Part model, mm, in its own coordinate system. Face numbers are marked on the shaded views. A direction names the side the tool comes from. Coordinates: 2 decimals unless noted, no trailing zeros. Loops run counter-clockwise (first coordinate to the right, second up) from the corner with the lowest first, then second, coordinate; pieces in that order, holes last. Notation, with made-up numbers: (29, 60) -> (52, 60) arc R22 cw to (52, 99) -> close; hole circle Ø5 at (-15.5, 8). An arc over 180 degrees is marked (long way). One line per question, with ' | ' between items. Start each with the question number.
1) Two-plate mould, pull along X, no slides. Class the marked faces 4, 5, 6 and 7: released by +X, released by -X, zero draft, split by the parting line, or undercut.
2) 3-axis set-ups, long thin cutter, end or side, ignore diameter. For the marked faces 1, 2 and 3: which of +Z, -Z, +X, -X, +Y, -Y reach the whole face in a straight line?
3) Cut at A-A (z = 45). List the corners of the cut face in (x, y), plus the area to 3 significant figures.
4) Cut at B-B (x = -26). List the corners of the cut face in (y, z).
5) Drop flat-ended pins along their axis: pin 1 (8 mm diameter, centred on y = -10, z = 50, fed in from +X); pin 2 (10.5 mm diameter, centred on x = 5, z = 18.5, fed in from -Y); pin 3 (12 mm diameter, centred on x = -0.5, z = 28.5, fed in from +Y). Give the stop position or say it passes through.
6) Probe L1, parallel to X at y = -7.5, z = 21; L2, parallel to Y at x = 21.5, z = 33; L3, parallel to Y at x = 5, z = 51.5. List the from-to ranges inside material, lowest first. Write a range as from..to.
7) Cut at C-C (y = 20.5). List the corners of the cut face in (x, z).
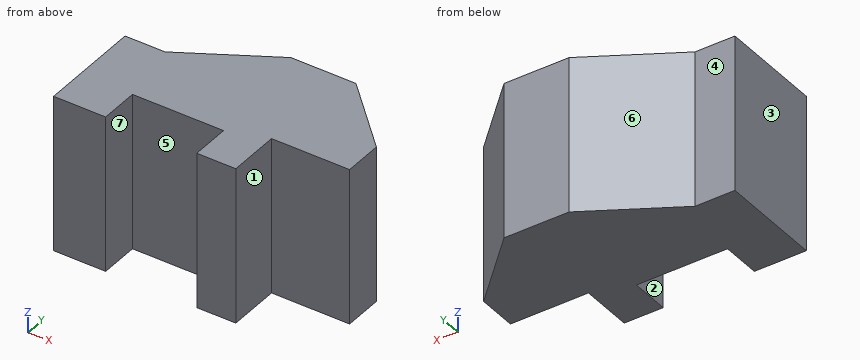
from build123d import *

# Parameters (mm, degrees)
F1_DEPTH = 60
F3_DEPTH = 25
F4_DEPTH = 78


with BuildPart() as f1:
    # F0 (on Top) → F1 (new body)
    with BuildSketch(Plane.XY):
        Polygon((66.599292, 42.537525), (-33.400708, 42.537525), (-33.400708, -17.462475), (-13.400708, -17.462475), (-13.400708, -2.462475), (21.599292, -2.462475), (21.599292, -17.462475), (36.599292, -17.462475), (36.599292, 2.537525), (66.599292, 2.537525), align=None)
    extrude(amount=F1_DEPTH)

    # F2 (on Top) → F3 (join)
    with BuildSketch(Plane.XY):
        Polygon((66.599292, 17.537525), (66.599292, 42.537525), (41.599292, 42.537525), align=None)
        Polygon((16.599292, 42.537525), (-33.400708, 42.537525), (-33.400708, 23.578404), (-33.400708, 22.537525), (-18.041724, 22.537525), align=None)
    extrude(amount=F3_DEPTH)

    # F2 (on Top) → F4 (cut)
    with BuildSketch(Plane.XY):
        Polygon((66.599292, 17.537525), (66.599292, 42.537525), (41.599292, 42.537525), align=None)
        Polygon((16.599292, 42.537525), (-33.400708, 42.537525), (-33.400708, 23.578404), (-33.400708, 22.537525), (-18.041724, 22.537525), align=None)
    extrude(amount=F4_DEPTH, mode=Mode.SUBTRACT)


solid = f1.part
Reported:
1) face 4: zero draft | face 5: undercut | face 6: released by -X | face 7: undercut
2) face 1: +Z, -Z, +X, -Y | face 2: +Z, -Z, -Y | face 3: +Z, -Z, -X, +Y, -Y
3) outline: (-33.4, -17.46) -> (-13.4, -17.46) -> (-13.4, -2.46) -> (21.6, -2.46) -> (21.6, -17.46) -> (36.6, -17.46) -> (36.6, 2.54) -> (66.6, 2.54) -> (66.6, 17.54) -> (41.6, 42.54) -> (16.6, 42.54) -> (-18.04, 22.54) -> (-33.4, 22.54) -> close | area: 3,910 mm²
4) outline: (-17.46, 0) -> (22.54, 0) -> (22.54, 60) -> (-17.46, 60) -> close
5) pin 1: stops at x = 36.6 | pin 2: stops at y = -2.46 | pin 3: stops at y = 36.13
6) L1: x = -33.4..-13.4, 21.6..36.6 | L2: y = -2.46..42.54 | L3: y = -2.46..35.84
7) outline: (-33.4, 0) -> (63.64, 0) -> (63.64, 60) -> (-33.4, 60) -> close
